Check sheet for the modelled part. Datum: model origin and axes. Units: mm. Face numbers are marked on the shaded views. Round coordinates to 2 decimals unless told otherwise and drop trailing zeros. Order: outer loops, then holes, each group sorted by start corner. A loop starts at its lowest first (then second) coordinate and runs counter-clockwise, first axis right, second up. Notation, with made-up numbers: (59, 51) -> (92, 51) arc R17 ccw to (92, 74) -> close; hole circle Ø11 at (44.25, 64). An arc over 180 degrees is marked (long way). Answer in a Markdown table with one row per item.
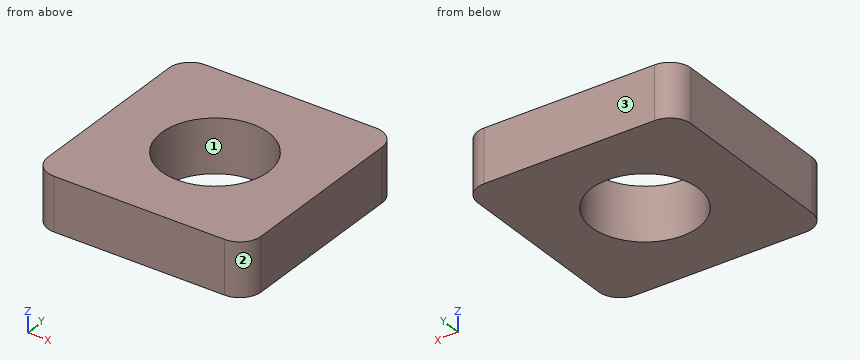
Autodesk Inventor part; units mm, degrees
ref_plane "YZ Plane" through (0, 0, 0) normal (1, 0, 0) x (0, 1, 0)
ref_plane "XZ Plane" through (0, 0, 0) normal (0, 1, 0) x (-1, 0, 0)
ref_plane "XY Plane" through (0, 0, 0) normal (0, 0, 1) x (1, 0, 0)
sketch "スケッチ1" plane through (0, 0, 0) normal (0, 0, 1) x (1, 0, 0)
  line L0 (-10, 10) -> (10, 10)
  line L1 (10, 10) -> (10, -10)
  line L2 (10, -10) -> (-10, -10)
  line L3 (-10, -10) -> (-10, 10)
  point P0 (0, 0)
  dimension "d0" = 20
  dimension "d1" = 20
  dimension "d2" = 10
  dimension "d3" = 10
extrude "押し出し1" add sketch "スケッチ1" along normal blind 5
sketch "スケッチ2" plane through (0, 0, 0) normal (0, 0, 1) x (1, 0, 0)
  circle A0 centre (0, 0) radius 5
  dimension "d6" = 10
extrude "押し出し2" cut sketch "スケッチ2" along normal blind 5
fillet "フィレット1" radius 2 4 edges at (10, 10, 2.5) (10, -10, 2.5) (-10, -10, 2.5) (-10, 10, 2.5)
properties part number "HbSensorCushion02" material "ゴム"
Item 1: Cross-section at C-C (z = 1.25). Record the boundary of the cut face in (x, y), and give its area (3 significant figures).
Result sheet:
| item | result |
|---|---|
| outline | (-10, -8) arc R2 ccw to (-8, -10) -> (8, -10) arc R2 ccw to (10, -8) -> (10, 8) arc R2 ccw to (8, 10) -> (-8, 10) arc R2 ccw to (-10, 8) -> close; hole circle Ø10 at (0, 0) |
| area | 318 mm^2 |
Item 2: Mould release check, pull along X, two halves, no side actions. Record for the marked faces 1, 2 and 3: pulls with the +X half, pulls with the -X half, needs draft (parallel to the pull), parting line crosses it, or undercut.
Result sheet:
| item | result |
|---|---|
| face 1 | undercut |
| face 2 | pulls with the +X half |
| face 3 | needs draft |
Item 3: Scan lines: line 1 (Y direction, x = 0, z = 3.65); line 2 (X direction, y = -3, z = 0.7); line 3 (Y direction, x = 2, z = 2). Record each from-to range of solid material in increasing order. Write a range as [from, to].
Result sheet:
| item | result |
|---|---|
| line 1 | y = [-10, -5], [5, 10] |
| line 2 | x = [-10, -4], [4, 10] |
| line 3 | y = [-10, -4.58], [4.58, 10] |
Item 4: Cross-section at A-A (x = 0). Record the boundary of the cut face in (y, z).
Result sheet:
| item | result |
|---|---|
| outline | (-10, 0) -> (-5, 0) -> (-5, 5) -> (-10, 5) -> close; (5, 0) -> (10, 0) -> (10, 5) -> (5, 5) -> close |
Item 5: Depth check by flat-ended pin: P1, Ø6, axis at x = 0, y = 0, coming from the -Z side. Enter the tip coordinate at first touch or a pass-through.
Result sheet:
| item | result |
|---|---|
| P1 | passes through |
